```python
from build123d import *

# Parameters (mm, degrees)
BOSS_EXTRUDE1_DEPTH = 19
CUT_EXTRUDE1_DEPTH  = 9.75
SKETCH5_R           = 2
CUT_EXTRUDE3_DEPTH  = 55.954526656
BOSS_EXTRUDE3_DEPTH = 3
CUT_EXTRUDE4_DEPTH  = 53.535702146
CUT_EXTRUDE6_START  = -7
CUT_EXTRUDE6_DEPTH  = 33.5
FILLET1_R           = 4
CHAMFER2_SIZE       = 2


with BuildPart() as part:
    # Sketch1 → Boss-Extrude1 (new, symmetric)
    with BuildSketch(Plane(origin=(0, 0, 0), x_dir=(0, 0, -1), z_dir=(1, 0, 0))):
        Polygon((-10, -12), (-10, -26), (6.666666667, -26), (30, 2), (30, 12), (10, 12), align=None)
    extrude(amount=BOSS_EXTRUDE1_DEPTH, both=True)

    # Sketch2 → Cut-Extrude1 (cut, symmetric)
    with BuildSketch(Plane(origin=(0, 0, 0), x_dir=(0, 0, -1), z_dir=(1, 0, 0))):
        Polygon((30, 6), (10, 6), (10, 12), (-4, 12), (-4, 6), (-10, 6), (-10, -12), (-4, -12), (-4, -26), (30, -26), align=None)
    extrude(amount=CUT_EXTRUDE1_DEPTH, both=True, mode=Mode.SUBTRACT)

    # Sketch5 → Cut-Extrude3 (cut, through all)
    with BuildSketch(Plane(origin=(19, 0, 0), x_dir=(0, 0, -1), z_dir=(1, 0, 0))):
        with Locations((18, -3)):
            Circle(SKETCH5_R)
    extrude(amount=-CUT_EXTRUDE3_DEPTH, mode=Mode.SUBTRACT)

    # Sketch6 → Boss-Extrude3 (add)
    with BuildSketch(Plane(origin=(19, 0, 0), x_dir=(0, 0, -1), z_dir=(1, 0, 0))):
        Polygon((18.177341601, 12), (25.409256694, -3.508891967), (30, 2), (30, 12), align=None)
    boss_extrude3 = extrude(amount=BOSS_EXTRUDE3_DEPTH)

    # Sketch7 → Cut-Extrude4 (cut, through all)
    with BuildSketch(Plane.XY.offset(10)):
        Polygon((-9.75, -12), (-4.75, -17), (4.75, -17), (9.75, -12), align=None)
    extrude(amount=-CUT_EXTRUDE4_DEPTH, mode=Mode.SUBTRACT)

    # Mirror2: Boss-Extrude3 across plane
    add(boss_extrude3.mirror(Plane(origin=(0, 0, 0), x_dir=(0, 0, 1), z_dir=(1, 0, 0))))

    # Sketch9 → Cut-Extrude6 (cut)
    with BuildSketch(Plane(origin=(-9.75, 0, 0), x_dir=(0, 0, -1), z_dir=(1, 0, 0)).offset(CUT_EXTRUDE6_START)):
        Polygon((13.958548116, -3), (15.979274058, -6.5), (20.020725942, -6.5), (22.041451884, -3), (20.020725942, 0.5), (15.979274058, 0.5), align=None)
    extrude(amount=CUT_EXTRUDE6_DEPTH, mode=Mode.SUBTRACT)

    # Fillet1
    fillet1_edges = [part.edges().sort_by_distance(p)[0] for p in [
        (22, 7, -30),
        (19, -19, 10),
        (-19, -19, 10),
        (-22, 7, -30),
    ]]
    fillet(fillet1_edges, radius=FILLET1_R)

    # Chamfer2
    # the kernel refuses this chamfer: 2 mm, written as the material it takes off along each edge
    with BuildSketch(Plane(origin=(-9.75, -15.951243191, 13.29270266), x_dir=(-0.9996219169112968, 0.017602431261197007, 0.02112291751343641), z_dir=(0, 0.7682212795973759, -0.6401843996644799))) as chamfer2_piece_1_section:
        Polygon((CHAMFER2_SIZE * 0.999621916911, -CHAMFER2_SIZE * 0.0274958766106), (-CHAMFER2_SIZE * 0.0274958766106, -CHAMFER2_SIZE * 0.999621916911), (0, 0), align=None)
    chamfer2_piece_1 = extrude(amount=41.527730655, mode=Mode.PRIVATE)
    chamfer2_piece_1 = split(chamfer2_piece_1, bisect_by=Plane(origin=(-15.992155631, -5.757844369, -0.703880227), z_dir=(0.7071067811865478, 0.7071067811865474, 0)), keep=Keep.TOP, mode=Mode.PRIVATE)
    chamfer2_piece_1 = split(chamfer2_piece_1, bisect_by=Plane(origin=(-10.414483767, -0.180172505, -10), z_dir=(0, 0, 1)), keep=Keep.TOP, mode=Mode.PRIVATE)
    add(chamfer2_piece_1, mode=Mode.SUBTRACT)
    with BuildSketch(Plane(origin=(-9.75, -29.951243191, -3.373964007), x_dir=(0.02749587661058651, 0.639942356769315, 0.7679308281231783), z_dir=(0, 0.768221279597376, -0.6401843996644798))) as chamfer2_piece_2:
        Polygon((CHAMFER2_SIZE * 0.999621916911, -CHAMFER2_SIZE * 0.0274958766106), (-CHAMFER2_SIZE * 0.0274958766106, -CHAMFER2_SIZE * 0.999621916911), (0, 0), align=None)
    extrude(amount=46.734563773, mode=Mode.SUBTRACT)
    with BuildSketch(Plane(origin=(9.75, -15.951243191, 13.29270266), x_dir=(0.9996219169112968, 0.017602431261197007, 0.02112291751343641), z_dir=(0, 0.7682212795973759, -0.6401843996644799))) as chamfer2_piece_3_section:
        Polygon((CHAMFER2_SIZE * 0.999621916911, CHAMFER2_SIZE * 0.0274958766106), (-CHAMFER2_SIZE * 0.0274958766106, CHAMFER2_SIZE * 0.999621916911), (0, 0), align=None)
    chamfer2_piece_3 = extrude(amount=41.527730655, mode=Mode.PRIVATE)
    chamfer2_piece_3 = split(chamfer2_piece_3, bisect_by=Plane(origin=(15.992155631, -5.757844369, -0.703880227), z_dir=(-0.7071067811865477, 0.7071067811865475, 0)), keep=Keep.TOP, mode=Mode.PRIVATE)
    chamfer2_piece_3 = split(chamfer2_piece_3, bisect_by=Plane(origin=(10.414483767, -0.180172505, -10), z_dir=(0, 0, 1)), keep=Keep.TOP, mode=Mode.PRIVATE)
    add(chamfer2_piece_3, mode=Mode.SUBTRACT)
    with BuildSketch(Plane(origin=(9.75, 5.951243191, -33.29270266), x_dir=(0.9996219169112968, -0.017602431261197003, -0.02112291751343641), z_dir=(0, -0.768221279597376, 0.6401843996644798))) as chamfer2_piece_4:
        Polygon((CHAMFER2_SIZE * 0.999621916911, CHAMFER2_SIZE * 0.0274958766106), (-CHAMFER2_SIZE * 0.0274958766106, CHAMFER2_SIZE * 0.999621916911), (0, 0), align=None)
    extrude(amount=46.734563773, mode=Mode.SUBTRACT)


solid = part.part
```
Here's how the part is built. I have some questions about the finished solid (model axes, mm). A direction names the side the tool comes from. Round coordinates to 2 decimals unless told otherwise and drop trailing zeros. Order: outer loops, then holes, each group sorted by start corner. A loop starts at its lowest first (then second) coordinate and runs counter-clockwise, first axis right, second up. Notation, with made-up numbers: M -32,-39 L 2,-39 A19 ccw 2,-21 Z; hole C 39.5,-21.5 d2. An arc over 180 degrees is marked long. Use CSV: the item, a comma, the result in double quotes.
1) I want a section at B-B (y = 4.5). List the corners of the cut face in (x, z) for me.
Taken from the geometry:
outline,"M -22,-26 A4 ccw -18,-30 L -10.15,-30 L -9.75,-29.48 L -9.75,-6.35 L -11.75,-3.75 L -19,-3.75 L -19,-21.67 L -22,-21.67 Z; M 9.75,-29.48 L 10.15,-30 L 18,-30 A4 ccw 22,-26 L 22,-21.67 L 19,-21.67 L 19,-3.75 L 11.75,-3.75 L 9.75,-6.35 Z"
2) I want a section at C-C (z = -1). List the corners of the cut face in (x, y) for me.
Taken from the geometry:
outline,"M -19,-26 L -9.75,-26 L -9.75,-1.92 L -11.75,1.2 L -19,1.2 Z; M 9.75,-26 L 19,-26 L 19,1.2 L 11.75,1.2 L 9.75,-1.92 Z"
3) I want a section at D-D (x = -9). List the corners of the cut face in (y, z) for me.
Taken from the geometry:
outline,"M -26,4 L -12.75,4 L -12.75,10 L -26,10 Z; M 6,-30 L 12,-30 L 12,-10 L 6,-10 Z"
4) I want a section at A-A (x = 3.5). List the corners of the cut face in (y, z) for me.
Taken from the geometry:
outline,"M -26,4 L -17,4 L -17,10 L -26,10 Z; M 6,-30 L 12,-30 L 12,-10 L 6,-10 Z"
5) If we mould it in two halves opening along Y, with no side actions, what happens to faces 1 (the flat face through (20.479, 4.354, -21.743)), 2 (the flat face through (0, 12, -20)), 3 (the flat face through (13.201, -1.274, -21.045))? For each: pulls with the +Y half, pulls with the -Y half, needs draft (parallel to the pull), parting line crosses it, or undercut.
Taken from the geometry:
face 1,"pulls with the -Y half"
face 2,"pulls with the +Y half"
face 3,"undercut"
6) I need wall thicknesses on line 1 along X through (y, z) = (-1.5, -9); line 2 along Y through (x, z) = (-8, -23). Which ranges of each line are inside material? Lowest first, please. Write a range as [from, to].
Taken from the geometry:
line 1,"[-19, -9.75], [9.75, 19]"
line 2,"[6, 12]"
7) I'm going to push flat-ended pins straight in: P1, Ø12, axis at y = -10, z = -25, coming from the +X side; P2, Ø3, axis at x = 1, y = 9.5, coming from the +Z side; P3, Ø10, axis at y = -3.5, z = -14, coming from the -X side; P4, Ø3.5, axis at y = -3, z = -18, coming from the -X side. Where does each tip first touch, or does it pass through?
Taken from the geometry:
P1,"x = 19"
P2,"z = -10"
P3,"x = -19"
P4,"through"
8) On a 3-axis mill with a long thin cutter (end or side, diameter ignored), from which of +Z, -Z, +X, -X, +Y, -Y can I reach the whole of each face in a straight line? I mean faces 4 (the flat face through (10.764, -10.869, -17.992)), 5 (the flat face through (-10.764, -0.15, -1.158)), 6 (the flat face through (13, 0.5, -18)). Say none if no direction works.
Taken from the geometry:
face 4,"-Z, -Y"
face 5,"+Z, +Y"
face 6,"none"
